Here's how the part is built. I have some questions about the finished solid (model axes, mm). A direction names the side the tool comes from. Give positions to 0.01 mm unless a question says otherwise; leave off trailing zeros. Loops run counter-clockwise (first coordinate to the right, second up) from the corner with the lowest first, then second, coordinate; pieces in that order, holes last.
Q1. If we section it at B-B (y = 3): Please give me the cut outline in (x, z), plus the area to 3 significant figures.
Q2. Will these pins go through, and if not, where does the flat tip stop? P1, Ø6, axis at x = 3, y = -17, coming from the +Z side; P2, Ø5, axis at x = 29.5, z = 7.5, coming from the -Y side.
Q3. If we section it at C-C (z = 4.5): Please give me the cut outline in (x, y), plus the area to 3 significant figures.
Q4. I need wall thicknesses on line 1 (Z direction, x = -26, y = -12); line 2 (Y direction, x = 40, z = 22.5). Which ranges of each line are inside material? Lowest first, please.
Q5. For faces 1 (the face through (1, 59, 57)), 2 (the face through (1, 57, 29)), which set-ups out of +Z, -Z, +X, -X, +Y, -Y let a thin tool reach every point of the face, with its end or its side?
Q6. If we section it at A-A (x = 11): Please give me the cut outline in (y, z).
from build123d import *

# Parameters (mm, degrees)
SKETCH_1_W                       = 100
SKETCH_1_H                       = 120
SM_BASE_FLANGE_1_DEPTH           = 3
SM_EDGE_FLANGE_1_STRIP_W         = 13.4732
SM_EDGE_FLANGE_1_STRIP_H         = 3
SM_EDGE_FLANGE_1_STRIP_CUT_DEPTH = 100
SM_EDGE_FLANGE_1_DEPTH           = 100


# Sheet-metal steps are written as plain solids
with BuildPart() as part:
    # Sketch 1 → 基体-法兰1 (new body)
    with BuildSketch(Plane.XY):
        Rectangle(SKETCH_1_W, SKETCH_1_H)
    extrude(amount=-SM_BASE_FLANGE_1_DEPTH)

    # 边线-法兰1 strip (across the edge) → 边线-法兰1 strip cut (cut)
    with BuildSketch(Plane(origin=(50, 60, 0), x_dir=(0, -1, 0), z_dir=(-1, 0, 0))):
        with Locations((-3, -1.5)):
            Rectangle(SM_EDGE_FLANGE_1_STRIP_W, SM_EDGE_FLANGE_1_STRIP_H)
    extrude(amount=SM_EDGE_FLANGE_1_STRIP_CUT_DEPTH, mode=Mode.SUBTRACT)

    # 边线-法兰1 section (across the edge) → 边线-法兰1 (add)
    with BuildSketch(Plane(origin=(50, 60, 0), x_dir=(0, -1, 0), z_dir=(-1, 0, 0))):
        with BuildLine():
            Line((0, 0.7366), (0, 57))
            Line((0, 57), (3, 57))
            Line((3, 57), (3, 0.7366))
            ThreePointArc((3, 0.7366), (3.215745145, 0.215745145), (3.7366, 0))
            Line((3.7366, 0), (3.7366, -3))
            ThreePointArc((3.7366, -3), (1.094424801, -1.905575199), (0, 0.7366))
        make_face()
    extrude(amount=SM_EDGE_FLANGE_1_DEPTH)


solid = part.part
Check sheet entries:
1. outline: (-50, -3) - (50, -3) - (50, 0) - (-50, 0) - close
1. area: 300 mm2
2. P1: stops at z = 0
2. P2: stops at y = 57
3. outline: (-50, 57) - (50, 57) - (50, 60) - (-50, 60) - close
3. area: 300 mm2
4. line 1: z = -3 to 0
4. line 2: y = 57 to 60
5. face 1: +Z, +X, -X, +Y, -Y
5. face 2: +Z, +X, -X, -Y
6. outline: (-60, -3) - (56.26, -3) arc R3.74 ccw to (60, 0.74) - (60, 57) - (57, 57) - (57, 0.74) arc R0.74 cw to (56.26, 0) - (-60, 0) - close
